Input: part model. Units: mm. Frame: model coordinates. A direction names the side the tool comes from. Round coordinates to 2 decimals unless told otherwise and drop trailing zeros. One line per question, with ' | ' between items.
Autodesk Inventor part; units mm, degrees
ref_plane "Work Plane1" through (-152.4, 0, 0) normal (-1, 0, 0) x (0, 0, 1)
ref_plane "YZ Plane" through (0, 0, 0) normal (1, 0, 0) x (0, 1, 0)
ref_plane "XZ Plane" through (0, 0, 0) normal (0, 1, 0) x (-1, 0, 0)
sketch "Sketch1" plane through (0, 0, 0) normal (0, 1, 0) x (-1, 0, 0)
  line L0 (0, 0) -> (304.8, 0)
  line L1 (304.8, 0) -> (304.8, 152.4)
  line L2 (304.8, 152.4) -> (0, 152.4)
  line L3 (0, 152.4) -> (0, 0)
  dimension "d0" = 304.8
  dimension "d1" = 152.4
extrude "Extrusion1" add sketch "Sketch1" along normal blind 12.7
hole "Hole1" at (-114.3, 12.7, 76.2) direction (0, -1, 0) diameter 0.508 end through all
hole "Hole2" at (-50.8, 12.7, 76.2) direction (0, -1, 0) diameter 0.508 end through all
hole "Hole3" at (-114.3, 0, 58.6994) direction (0, 1, 0) diameter 0.5 end through all countersink diameter 9.525 countersink angle 82
pattern_circular "Circular Pattern1" count 4 over 360 about axis through (-114.3, -328.3133, 76.2) along (0, 1, 0) of "Hole3"
sketch "Sketch4" plane through (0, 12.7, 0) normal (0, 1, 0) x (1, 0, 0)
  circle A0 centre (-114.3, -76.2) radius 0.254
  circle A1 centre (-114.3, -76.2) radius 12.0332
  dimension "d41" = 24.0665
sketch "Sketch5" plane through (0, 12.7, 0) normal (0, 1, 0) x (1, 0, 0)
  circle A0 centre (-50.8, -76.2) radius 0.254
  circle A1 centre (-114.3, -76.2) radius 0.254
  line L0 (0, 0) -> (-304.8, 0)
  line L1 (-304.8, 0) -> (-304.8, -152.4)
  line L2 (-304.8, -152.4) -> (0, -152.4)
  line L3 (0, -152.4) -> (0, 0)
  circle A2 centre (-114.3, -76.2) radius 22.5425
  dimension "d42" = 45.085
extrude "Extrusion4" add sketch "Sketch5" along normal blind 6.35 contours L3 L2 L1 L0
extrude "Extrusion5" cut sketch "Sketch4" against normal blind 2.032
hole "Hole4" at (-26.9748, 0, 76.2) direction (0, 1, 0) diameter 0.508 end through all countersink diameter 9.525 countersink angle 82
pattern_circular "Circular Pattern2" count 6 over 360 about axis through (-50.8, 19.05, 76.2) along (0, -1, 0) of "Hole4"
hole "Hole5" at (0, 9.525, 114.3) direction (-1, 0, 0) diameter 3.9624 depth 38.1 tip angle 118
pattern_linear "Rectangular Pattern1" count 3 spacing 38.1 along (0, 0, -1) of "Hole5"
ref_plane "Work Plane1" through (-152.4, 0, 0) normal (-1, 0, 0) x (0, 0, 1)
mirror "Mirror1" about plane through (-152.4, 0, 0) normal (-1, 0, 0) of "Hole5", "Rectangular Pattern1"
properties part number "Traveler with pin point holes"
Item 1: First-contact query: pin 1 (3.5 mm diameter, centred on y = 9.525, z = 76.2, fed in from -X); pin 2 (3.5 mm diameter, centred on y = 9.525, z = 114.3, fed in from +X); pin 3 (3 mm diameter, centred on y = 9.525, z = 76.2, fed in from -X). Flat tips, straight axial feed; report the tip coordinate or a pass-through.
Report:
pin 1: x = -266.56 | pin 2: x = -38.24 | pin 3: x = -266.41
Item 2: Access query for faces 1 (the flat face through (-124, 12.7, 66)), 2 (the conical face through (-37.952, 3.709, 95.613)). Directions: +Z, -Z, +X, -X, +Y, -Y. A direction counts if a zero-diameter tool reaches every point of the face in a straight line with its end or side. Return the directions, or none.
Report:
face 1: +Y | face 2: -Y
Item 3: Line query: line 1 along Y through (x, z) = (-15, 76); line 2 along Z through (x, y) = (-285.5, 11.25); line 3 along Y through (x, z) = (-291, 114.3). Output: solid intervals per line, ascending. Write a range as from..to.
Report:
line 1: 0..7.55, 11.5..19.05 | line 2: 0..37.13, 39.07..75.23, 77.17..113.33, 115.27..152.4 | line 3: 0..7.54, 11.51..19.05
Item 4: Mould query, pull axis Z, two halves, no side actions, for faces 3 (the flat face through (-155, 19.05, 75)), 4 (the conical face through (-97.13, 3.71, 74.7)), 5 (the flat face through (-150, 9, 0)). Classes: +Z half, -Z half, draft (parallel to the pull), parting line (faces both ways), or undercut.
Report:
face 3: draft | face 4: undercut | face 5: -Z half
